CAD build for the part. Positions are in the model's coordinates, mm. A direction names the side the tool comes from. Coordinates: 2 decimals unless noted, no trailing zeros. Loops run counter-clockwise (first coordinate to the right, second up) from the corner with the lowest first, then second, coordinate; pieces in that order, holes last. Notation, with made-up numbers: (63.5, 63.5) -> (75.5, 63.5) arc R34 ccw to (75.5, 102.5) -> close; hole circle Ø5 at (53, 87). An arc over 180 degrees is marked (long way). Write each question's results on one line, items separated by ' | '.
Autodesk Inventor part; units mm, degrees
ref_plane "YZ Plane" through (0, 0, 0) normal (1, 0, 0) x (0, 1, 0)
ref_plane "XZ Plane" through (0, 0, 0) normal (0, 1, 0) x (-1, 0, 0)
ref_plane "XY Plane" through (0, 0, 0) normal (0, 0, 1) x (1, 0, 0)
sketch "スケッチ1" plane through (0, 0, 0) normal (0, 1, 0) x (-1, 0, 0)
  line L0 (-12.5, -15) -> (12.5, -15)
  line L1 (12.5, -15) -> (12.5, 15)
  line L2 (12.5, 15) -> (-12.5, 15)
  line L3 (-12.5, 15) -> (-12.5, -15)
  line L4 (-12.5, -15) -> (12.5, 15) construction
  line L5 (12.5, -15) -> (-12.5, 15) construction
  point P0 (0, 0)
  dimension "d0" = 25
  dimension "d1" = 30
extrude "押し出し1" add sketch "スケッチ1" along normal blind 25
sketch "スケッチ2" plane through (0, 0, 0) normal (0, -1, 0) x (1, 0, 0)
  line L0 (12.5, 15) -> (12.5, -15)
  line L1 (12.5, -10.25) -> (-8, -10.25)
  line L2 (-8, -10.25) -> (-8, 10.25)
  line L3 (-8, 10.25) -> (12.5, 10.25)
  line L4 (12.5, 10.25) -> (12.5, -10.25)
  line L5 (12.5, -15) -> (-12.5, -15)
  point P0 (0, 0)
  point P1 (12.5, 10.25)
  dimension "d4" = 20.5
  dimension "d5" = 20.5
  dimension "d22" = 10.25
extrude "押し出し2" cut sketch "スケッチ2" against normal blind 20
sketch "スケッチ4" plane through (12.5, 0, -15) normal (0, 0, -1) x (-1, 0, 0)
  line L0 (0, 0) -> (25, 0)
  line L1 (0, 0) -> (0, 25)
  point P0 (12.5, 0)
  point P1 (10.25, 7)
  dimension "d12" = 7
  dimension "d13" = 10.25
hole "穴1" at (2.25, 7, -15) direction (0, 0, 1) diameter 6 end through all
fillet "フィレット1" radius 0.5 8 edges at (12.5, 12.5, -15) (-12.5, 12.5, -15) (-12.5, 12.5, 15) (12.5, 12.5, 15) (12.5, 25, 0) (0, 25, -15) (-12.5, 25, 0) (0, 25, 15)
sketch "スケッチ5" plane through (0, 20, 0) normal (0, -1, 0) x (1, 0, 0)
  circle A0 centre (2.25, 0) radius 6.75
  line L0 (12.5, 10.25) -> (12.5, -10.25)
  line L1 (-8, 10.25) -> (12.5, 10.25)
  point P0 (0, 0)
  dimension "d24" = 13.5
  dimension "d25" = 10.25
  dimension "d26" = 10.25
extrude "押し出し4" cut sketch "スケッチ5" against normal blind 4
properties part number "baseA"
Q1. Cut at C-C on z = 0. Write the cut outline in (x, y), and give its area (3 significant figures).
Results are:
outline: (-12.5, 0) -> (-8, 0) -> (-8, 20) -> (-4.5, 20) -> (-4.5, 24) -> (9, 24) -> (9, 20) -> (12.5, 20) -> (12.5, 24.5) arc R0.5 ccw to (12, 25) -> (-12, 25) arc R0.5 ccw to (-12.5, 24.5) -> close | area: 161 mm^2
Q2. Cut at D-D on y = 7. Write the cut outline in (x, z).
Results are:
outline: (-12.5, -14.5) arc R0.5 ccw to (-12, -15) -> (-0.75, -15) -> (-0.75, -10.25) -> (-8, -10.25) -> (-8, 10.25) -> (-0.75, 10.25) -> (-0.75, 15) -> (-12, 15) arc R0.5 ccw to (-12.5, 14.5) -> close; (5.25, -15) -> (12, -15) arc R0.5 ccw to (12.5, -14.5) -> (12.5, -10.25) -> (5.25, -10.25) -> close; (5.25, 10.25) -> (12.5, 10.25) -> (12.5, 14.5) arc R0.5 ccw to (12, 15) -> (5.25, 15) -> close
Q3. Which spindle directions (+Z, -Z, +X, -X, +Y, -Y) get a long thin tool onto all of the face, cutting with end or side? Do faces 4 (the flat face through (2, 24, 0)), 5 (the flat face through (-8.2, 0, 0.2)), 6 (the flat face through (-8, 10, 0)). Say none if no direction does.
Results are:
face 4: -Y | face 5: +Z, -Z, +X, -X, -Y | face 6: +X, -Y
Q4. Drop flat-ended pins along their axis: pin 1 (4 mm diameter, centred on x = -9.5, z = -8, fed in from -Y); pin 2 (11 mm diameter, centred on x = 5.5, z = 1, fed in from -Y). Give the stop position or say it passes through.
Results are:
pin 1: y = 0 | pin 2: y = 20
Q5. Wall check: L1, parallel to X at y = 7, z = -12.5; L2, parallel to Z at x = 7, y = 11.75; L3, parallel to Z at x = 2.25, y = 22.3. Give the ranges that are in metal, low to high. Write a range as from..to.
Results are:
L1: -12.5..-0.75, 5.25..12.5 | L2: -15..-10.25, 10.25..15 | L3: -15..-6.75, 6.75..15
Q6. Cut at A-A on x = 2.25. Write the cut outline in (y, z).
Results are:
outline: (0, -15) -> (4, -15) -> (4, -10.25) -> (0, -10.25) -> close; (0, 10.25) -> (4, 10.25) -> (4, 15) -> (0, 15) -> close; (10, -15) -> (24.5, -15) arc R0.5 ccw to (25, -14.5) -> (25, 14.5) arc R0.5 ccw to (24.5, 15) -> (10, 15) -> (10, 10.25) -> (20, 10.25) -> (20, 6.75) -> (24, 6.75) -> (24, -6.75) -> (20, -6.75) -> (20, -10.25) -> (10, -10.25) -> close
Q7. Pull direction Z, two halves, no side cores. Call faces 1 (the flat face through (0, 12, 15)), 2 (the flat face through (2, 12, 10.25)), 3 (the flat face through (-12.5, 12, 0)): +Z half, -Z half, draft (parallel to the pull), parting line (faces both ways), or undercut.
Results are:
face 1: +Z half | face 2: undercut | face 3: draft
Q8. Cut at B-B on y = 20.75. Write the cut outline in (x, z), and give its area (3 significant figures).
Results are:
outline: (-12.5, -14.5) arc R0.5 ccw to (-12, -15) -> (12, -15) arc R0.5 ccw to (12.5, -14.5) -> (12.5, 14.5) arc R0.5 ccw to (12, 15) -> (-12, 15) arc R0.5 ccw to (-12.5, 14.5) -> close; hole circle Ø13.5 at (2.25, 0) | area: 607 mm^2
